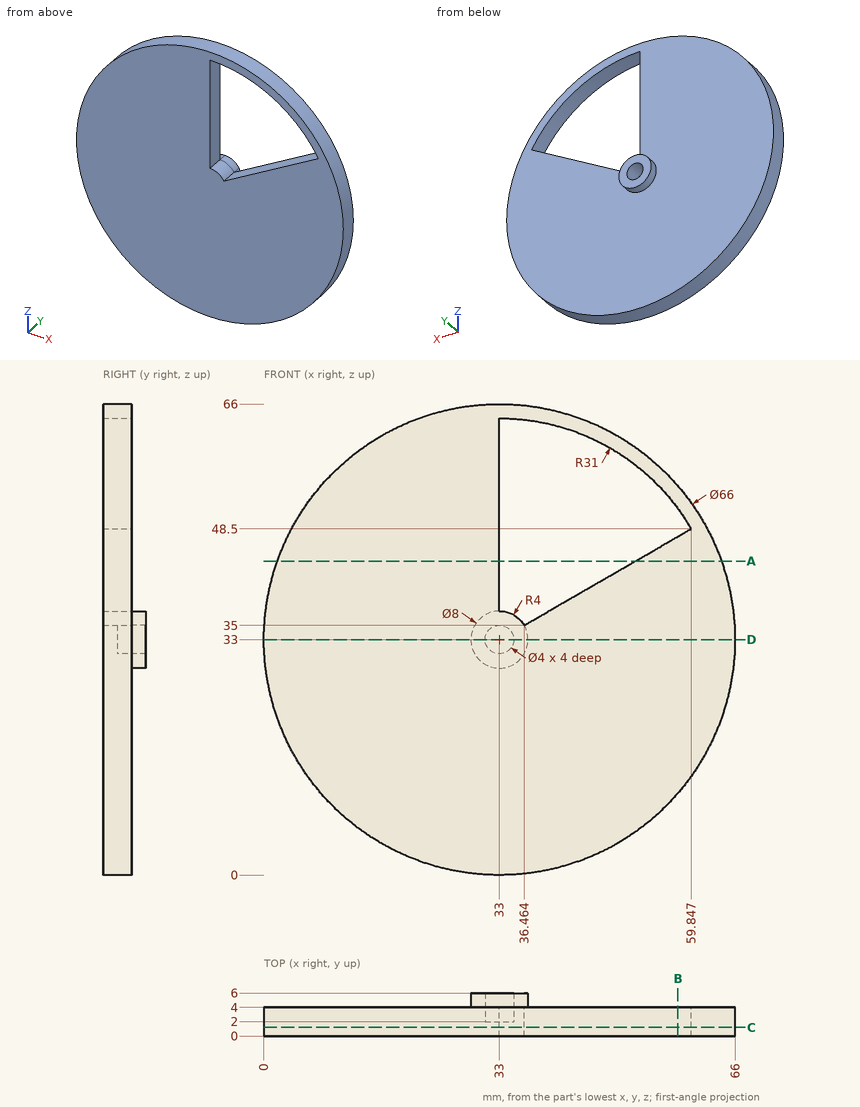
Design review of the part shown in the three views and the two pictorial views. Dimensions are in mm from the part's minimum x, y and z. Round coordinates to 2 decimals unless told otherwise and drop trailing zeros. Loops run counter-clockwise (first coordinate to the right, second up) from the corner with the lowest first, then second, coordinate; pieces in that order, holes last. Notation, with made-up numbers: M -33.75,66 L -1.75,66 A18 ccw -1.75,73 Z; hole C 20.25,65 d9. An arc over 180 degrees is marked long. Answer as a JSON object with one key per item and string values.
Item 1: We need section D-D, the plane z = 33. State the section outline as (x, y) points, and give its area (3 significant figures).
Check sheet entries:
{"outline": "M 0,0 L 66,0 L 66,4 L 37,4 L 37,6 L 35,6 L 35,2 L 31,2 L 31,6 L 29,6 L 29,4 L 0,4 Z", "area": "264 mm2"}
Item 2: We need section C-C, the plane y = 1.2. State the section outline as (x, z) points, and give its area (3 significant figures).
Check sheet entries:
{"outline": "C 33,33 d66; hole M 33,37 A4 cw 36.46,35 L 59.85,48.5 A31 ccw 33,64 Z", "area": "2,930 mm2"}
Item 3: Clearance check with flat-ended pins moving along their axes: P1, Ø2, axis at x = 33.5, z = 32.5, coming from the +Y side; P2, Ø2, axis at x = 34.5, z = 57.5, coming from the +Y side; P3, Ø4, axis at x = 10.5, z = 57, coming from the +Y side; P4, Ø2, axis at y = 3, z = 19, coming from the +X side. State where each tip first meets the part, or that it passes through.
Check sheet entries:
{"P1": "y = 2", "P2": "through", "P3": "y = 4", "P4": "x = 63.33"}
Item 4: We need section A-A, the plane z = 44. State the section outline as (x, y) points, and give its area (3 significant figures).
Check sheet entries:
{"outline": "M 1.89,0 L 33,0 L 33,4 L 1.89,4 Z; M 52.05,0 L 64.11,0 L 64.11,4 L 52.05,4 Z", "area": "173 mm2"}
Item 5: We need section B-B, the plane x = 58. State the section outline as (y, z) points.
Check sheet entries:
{"outline": "M 0,11.46 L 4,11.46 L 4,47.43 L 0,47.43 Z; M 0,51.33 L 4,51.33 L 4,54.54 L 0,54.54 Z"}
Item 6: For line 1 along Y through (x, z) = (55, 21.5); line 2 along X through (y, z) = (2.8, 47); line 3 along X through (y, z) = (2.6, 58.5) (1 decimal), list the stretches that pass through material, from the lowest coordinate up.
Check sheet entries:
{"line 1": "0 to 4", "line 2": "3.12 to 33, 57.25 to 62.88", "line 3": "12.1 to 33, 50.6 to 53.9"}
